Autodesk Inventor part; units mm, degrees
ref_plane "YZ Plane" through (0, 0, 0) normal (1, 0, 0) x (0, 1, 0)
ref_plane "XZ Plane" through (0, 0, 0) normal (0, 1, 0) x (-1, 0, 0)
ref_plane "XY Plane" through (0, 0, 0) normal (0, 0, 1) x (1, 0, 0)
sketch "Sketch1" plane through (0, 0, 0) normal (0, 1, 0) x (-1, 0, 0)
  line L0 (10, -35) -> (-10, -35)
  line L1 (-10, -35) -> (-10, 44)
  line L2 (-10, 44) -> (10, 44)
  line L3 (10, 44) -> (10, -35)
  point P0 (0, 0)
  dimension "d0" = 20
  dimension "d1" = 79
  dimension "d2" = 35
  dimension "d3" = 10
extrude "Plate1" add sketch "Sketch1" along normal blind 1.5
sketch "Sketch3" plane through (0, 1.5, 0) normal (0, 1, 0) x (1, 0, 0)
  circle A0 centre (0, 25) radius 10
  circle A1 centre (0, -25) radius 10
  line L0 (-10, 35) -> (10, 35)
  line L1 (10, -44) -> (-10, -44)
  line L2 (-10, 35) -> (10, 35)
  line L3 (10, 35) -> (10, 25)
  line L4 (10, 25) -> (-10, 25)
  line L5 (-10, 25) -> (-10, 35)
  line L6 (10, -35) -> (-10, -35)
  line L7 (-10, -35) -> (-10, -25)
  line L8 (-10, -25) -> (10, -25)
  line L9 (10, -25) -> (10, -44)
  point P0 (0, 0)
  point P1 (10, -25)
  point P2 (0, -35)
  point P3 (-10, -35)
  point P4 (0, 35)
  point P5 (10, 35)
  dimension "d12" = 20
  dimension "d13" = 20
  dimension "d14" = 10
  dimension "d15" = 10
  dimension "d16" = 25
  dimension "d17" = 25
  dimension "d18" = 10
extrude "Extrusion1" cut sketch "Sketch3" against normal blind 10 contours L5 L0 A0 | A0 L0 L3
sketch "Sketch4" plane through (0, 1.5, 0) normal (0, 1, 0) x (1, 0, 0)
  circle A0 centre (-7, 25) radius 0.8
  arc A1 (10, 25) -> (-10, 25) centre (0, 25) ccw
  circle A2 centre (0, 18) radius 0.8
  circle A3 centre (7, 25) radius 0.8
  circle A4 centre (0, 32) radius 0.8
  point P0 (0, 0)
  dimension "d21" = 0
  dimension "d22" = 7
  dimension "d23" = 1.6
  dimension "d26" = 360
hole "Hole2" at (0, 1.5, -32) at (7, 1.5, -25) at (0, 1.5, -18) at (-7, 1.5, -25) direction (0, -1, 0) diameter 2.1 depth 1.5
equation "\"d33\" = Thickness"
equation "\"d4\" = Thickness"
equation "\"BendReliefWidth\" = Thickness"
equation "\"BendReliefDepth\" = 0.5 * Thickness"
equation "\"CornerReliefSize\" = 4 * Thickness"
equation "\"MinimumRemnant\" = 2 * Thickness"
equation "\"TransitionRadius\" = BendRadius"
equation "\"JacobiRadiusSize\" = BendRadius"
equation "\"GapSize\" = Thickness"
properties part number "axis_8_10_connector_frame" material "Aluminum 6061-AHC"
Input: part model. Units: mm. Frame: model coordinates. Coordinates: 2 decimals unless noted, no trailing zeros. Loops run counter-clockwise (first coordinate to the right, second up) from the corner with the lowest first, then second, coordinate; pieces in that order, holes last.
Q1. Cut plane D-D (z = -27). Output: boundary loops of the cut face in (x, y), then the cut area to 3 significant figures.
Q2. Cut plane A-A (z = -18). Output: boundary loops of the cut face in (x, y), then the cut area to 4 significant figures.
Q3. Cut plane B-B (y = 1.2). Output: boundary loops of the cut face in (x, z), then the cut area to 3 significant figures.
Q4. Draft query along X for faces 1 (the face through (0.4, 0.74, -31.03)), 2 (the face through (0, 1.5, 5)), 3 (the face through (0, 1, -35)). Return one class per face: +X half, -X half, draft (parallel to the pull), parting line (faces both ways), or undercut.
Q5. Cut plane C-C (x = 7). Output: boundary loops of the cut face in (y, z).
Q6. Material intervals for line 1 (Z direction, x = 0, y = 0.6); line 2 (X direction, y = 0.75, z = -25); line 3 (X direction, y = 0.9, z = -18), sorted ascending.
Working result:
1. outline: (-9.8, 0) - (9.8, 0) - (9.8, 1.5) - (-9.8, 1.5) - close
1. area: 29.4 mm2
2. outline: (-10, 0) - (-1.05, 0) - (-1.05, 1.5) - (-10, 1.5) - close; (1.05, 0) - (10, 0) - (10, 1.5) - (1.05, 1.5) - close
2. area: 26.85 mm2
3. outline: (-10, -25) arc R10 ccw to (10, -25) - (10, 44) - (-10, 44) - close; hole circle Ø2.1 at (-7, -25); hole circle Ø2.1 at (0, -32); hole circle Ø2.1 at (0, -18); hole circle Ø2.1 at (7, -25)
3. area: 1,520 mm2
4. face 1: undercut
4. face 2: draft
4. face 3: parting line
5. outline: (0, -32.14) - (1.5, -32.14) - (1.5, -26.05) - (0, -26.05) - close; (0, -23.95) - (1.5, -23.95) - (1.5, 44) - (0, 44) - close
6. line 1: z = -35 to -33.05, -30.95 to -19.05, -16.95 to 44
6. line 2: x = -10 to -8.05, -5.95 to 5.95, 8.05 to 10
6. line 3: x = -10 to -1.05, 1.05 to 10
